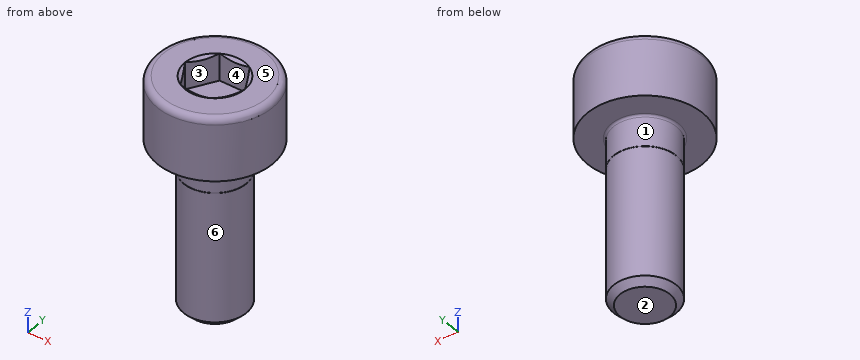
Solid Edge part; units mm, degrees
sketch "Sketch1" plane through (0, 0, 0) normal (0, 0, 1) x (1, 0, 0)
  circle A0 centre (0, 0) radius 2.75
extrude "Protrusion1" add sketch "Sketch1" along normal blind 3
sketch "Sketch2" plane through (0, 0, 3) normal (0, 0, 1) x (0, 1, 0)
  line L0 (0, 1.4434) -> (1.25, 0.7217)
  line L1 (1.25, 0.7217) -> (1.25, -0.7217)
  line L2 (1.25, -0.7217) -> (0, -1.4434)
  line L3 (0, -1.4434) -> (-1.25, -0.7217)
  line L4 (-1.25, -0.7217) -> (-1.25, 0.7217)
  line L5 (-1.25, 0.7217) -> (0, 1.4434)
extrude "Cutout1" cut sketch "Sketch2" against normal blind 1.3
fillet "Round1" radius 0.3 1 edges at (-2.75, 0, 3)
sketch "Sketch3" plane through (0, 0, 0) normal (1, 0, 0) x (0, 1, 0)
  line L0 (-1.1935, -8) -> (0, -8)
  line L1 (-1.5, -7.6935) -> (-1.1935, -8)
  line L2 (-1.5, -1.5) -> (-1.5, -7.6935)
  line L3 (-1.1935, -1.5) -> (-1.5, -1.5)
  line L4 (-1.1935, -1.49) -> (-1.1935, -1.5)
  line L5 (-1.5, -1.49) -> (-1.1935, -1.49)
  line L6 (-1.5, -0.1) -> (-1.5, -1.49)
  arc A0 (-1.5, -0.1) -> (-1.6, 0) centre (-1.6, -0.1) ccw
revolve "RevolvedProtrusion1" add sketch "Sketch3" angle 360 about axis through (0, 0, -60.325) along (0, 0, 1) material side at (0, -0.5968, -7.95)
cosmetic_thread "Thread1"
sketch "Sketch4" plane through (0, 0, 0) normal (0, -1, 0) x (1, 0, 0)
  line L0 (-1.435, 3) -> (0, 2.1715)
revolve "RevolvedCutout1" cut sketch "Sketch4" angle 360 about axis through (0, 0, 57.15) along (0, 0, -1) material side at (-0.6925, 0, 2.6291)
properties material "Stahl"
Here's how the part is built. I have some questions about the finished solid (model axes, mm). Face numbers are marked on the shaded views. A direction names the side the tool comes from. Round coordinates to 2 decimals unless told otherwise and drop trailing zeros. Loops run counter-clockwise (first coordinate to the right, second up) from the corner with the lowest first, then second, coordinate; pieces in that order, holes last. Notation, with made-up numbers: M 4.25,-7 L 9.25,-7 A13 cw 9.25,3 Z; hole C 47.5,65 d8. An arc over 180 degrees is marked long. Write each question's results on one line, items separated by ' | '. Start each with the question number.
(1) I want a section at B-B (z = 1). Please give me the cut outline in (x, y).
(2) Thinking about a two-plate mould opening in X: for the marked faces 4, 5 and 6, which applies, pulls with the +X half, pulls with the -X half, needs draft (parallel to the pull), parting line crosses it, or undercut?
(3) On a 3-axis mill with a long thin cutter (end or side, diameter ignored), from which of +Z, -Z, +X, -X, +Y, -Y can I reach the whole of each face in a straight line? I mean the marked faces 1, 2 and 3. Say none if no direction works.
(4) Will these pins go through, and if not, where does the flat tip stop? P1, Ø0.8, axis at x = 0.5, y = -0.5, coming from the +Z side; P2, Ø1, axis at x = 1.5, z = -3.5, coming from the -Y side; P3, Ø1, axis at x = -1.5, z = 0, coming from the +Y side.
(5) If I drill on probe 1 along Z at (x, y) = (1.7, 0.55); probe 2 along Y at (x, z) = (-0.1, -0.75); probe 3 along Z at (x, y) = (0.35, -0.6), over which ranges is the centre line in solid material (lowest first)? Write a range as from..to.
Solved:
1) outline: C 0,0 d5.5
2) face 4: undercut | face 5: needs draft | face 6: parting line crosses it
3) face 1: -Z | face 2: -Z, +X, -X, +Y, -Y | face 3: +Z
4) P1: stops at z = 1.7 | P2: stops at y = -1.12 | P3: stops at y = 2.56
5) probe 1: z = 0..3 | probe 2: y = -1.5..1.5 | probe 3: z = -8..1.7
